Autodesk Inventor part; units mm, degrees
ref_plane "YZ Plane" through (0, 0, 0) normal (1, 0, 0) x (0, 1, 0)
ref_plane "XZ Plane" through (0, 0, 0) normal (0, 1, 0) x (-1, 0, 0)
ref_plane "XY Plane" through (0, 0, 0) normal (0, 0, 1) x (1, 0, 0)
sketch "Эскиз1" plane through (0, 0, 0) normal (0, 1, 0) x (-1, 0, 0)
  circle A0 centre (0, 0) radius 1.4
  line L0 (0.8083, 1.4) -> (1.6166, 0)
  line L1 (1.6166, 0) -> (0.8083, -1.4)
  line L2 (0.8083, -1.4) -> (-0.8083, -1.4)
  line L3 (-0.8083, -1.4) -> (-1.6166, 0)
  line L4 (-1.6166, 0) -> (-0.8083, 1.4)
  line L5 (-0.8083, 1.4) -> (0.8083, 1.4)
  line L6 (0, 0) -> (3.2332, 0) construction
  dimension "d0" = 2.8
extrude "Выдавливание1" add sketch "Эскиз1" along normal blind 17
sketch "Эскиз2" plane through (0, 17, 0) normal (0, 1, 0) x (1, 0, 0)
  point P0 (0, 0)
  point P1 (0, 0)
hole "Отверстие1" at (0, 17, 0) direction (0, -1, 0) diameter 2.6 depth 4
sketch "Эскиз3" plane through (0, 0, 0) normal (0, -1, 0) x (1, 0, 0)
  circle A0 centre (0, 0) radius 1.2
  dimension "d10" = 2.4
extrude "Выдавливание2" add sketch "Эскиз3" along normal blind 3
properties part number "столбики"
CAD build for the part. Positions are in the model's coordinates, mm. A direction names the side the tool comes from. Round coordinates to 2 decimals unless told otherwise and drop trailing zeros. Order: outer loops, then holes, each group sorted by start corner. A loop starts at its lowest first (then second) coordinate and runs counter-clockwise, first axis right, second up. Notation, with made-up numbers: M 55.5,52 L 73.5,52 A28 cw 73.5,83 Z; hole C 50,-37.75 d10. An arc over 180 degrees is marked long. Use one line per item in the form item = value.
Q1. Probe L1, parallel to Y at x = -1.05, z = 0.7; L2, parallel to Y at x = -0.7, z = 0.2; L3, parallel to Z at x = 0.55, y = 15.5. List the from-to ranges inside material, lowest first.
Recorded:
L1 = 0 to 13
L2 = -3 to 13
L3 = -1.4 to -1.18, 1.18 to 1.4
Q2. Saw through at B-B on z = -0.45. Give the cut face in (x, y).
Recorded:
outline = M -1.36,0 L -1.11,0 L -1.11,-3 L 1.11,-3 L 1.11,0 L 1.36,0 L 1.36,17 L 1.22,17 L 1.22,13 L -1.22,13 L -1.22,17 L -1.36,17 Z
Q3. Which spindle directions (+Z, -Z, +X, -X, +Y, -Y) get a long thin tool onto all of the face, cutting with end or side? Do faces 1 (the flat face through (0, 8, 1.4)), 2 (the cylindrical face through (0.65, -1.48, -1.01)), 3 (the cylindrical face through (-1.29, 14.97, -0.17)). Say none if no direction does.
Recorded:
face_1 = +Z, +X, -X, +Y, -Y
face_2 = -Y
face_3 = +Y
Q4. Saw through at C-C on y = 9.25. Give the cut face in (x, z).
Recorded:
outline = M -1.62,0 L -0.81,-1.4 L 0.81,-1.4 L 1.62,0 L 0.81,1.4 L -0.81,1.4 Z
Q5. Two-plate mould, pull along Z, no slides. Class faces 4 (the flat face through (0, 13, 0)), 5 (the flat face through (0, -3, 0)), 6 (the flat face through (-1.22, 8.38, -0.69)): +Z half, -Z half, draft (parallel to the pull), parting line (faces both ways), or undercut.
Recorded:
face_4 = undercut
face_5 = draft
face_6 = -Z half
Q6. Saw through at D-D on y = -1. Give the cut face in (x, z), then the cut area to 3 significant figures.
Recorded:
outline = C 0,0 d2.4
area = 4.52 mm^2
Q7. Saw through at A-A on x = -0.45. Give the cut face in (y, z), then the cut area to 3 significant figures.
Recorded:
outline = M -3,-1.11 L 0,-1.11 L 0,-1.4 L 17,-1.4 L 17,-1.22 L 13,-1.22 L 13,1.22 L 17,1.22 L 17,1.4 L 0,1.4 L 0,1.11 L -3,1.11 Z
area = 44.5 mm^2
